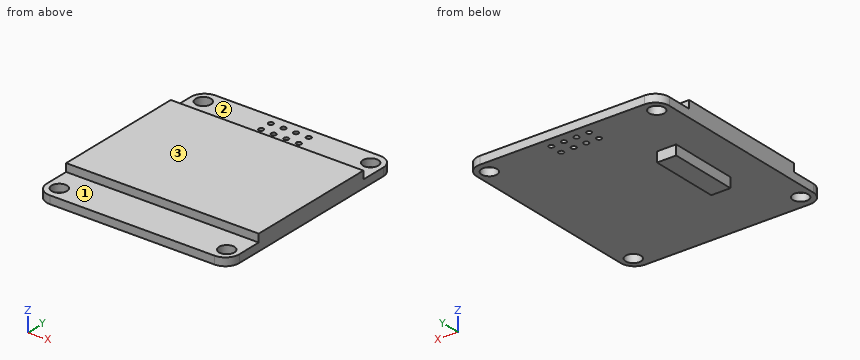
from build123d import *

# Parameters (mm, degrees)
SKIZZE1_R                       = 1.55
AUFSATZ_LINEAR_AUSTRAGEN1_DEPTH = 1.6
SKIZZE2_R                       = 0.5
SCHNITT_LINEAR_AUSTRAGEN1_DEPTH = 1.6
SKIZZE3_W                       = 38.8
SKIZZE3_H                       = 27.043851976
AUFSATZ_LINEAR_AUSTRAGEN2_DEPTH = 1.6
SKIZZE4_W                       = 3.86922581
SKIZZE4_H                       = 14.010670301
AUFSATZ_LINEAR_AUSTRAGEN3_DEPTH = 2


with BuildPart() as part:
    # Skizze1 → Aufsatz-Linear austragen1 (new body)
    with BuildSketch(Plane.XY):
        with BuildLine():
            Line((16.6, -21.4), (-16.6, -21.4))
            ThreePointArc((-16.6, -21.4), (-18.579898987, -20.579898987), (-19.4, -18.6))
            Line((-19.4, -18.6), (-19.4, 18.6))
            ThreePointArc((-19.4, 18.6), (-18.579898987, 20.579898987), (-16.6, 21.4))
            Line((-16.6, 21.4), (16.6, 21.4))
            ThreePointArc((16.6, 21.4), (18.579898987, 20.579898987), (19.4, 18.6))
            Line((19.4, 18.6), (19.4, -18.6))
            ThreePointArc((19.4, -18.6), (18.579898987, -20.579898987), (16.6, -21.4))
        make_face()
        with Locations((-16.861682243, 18.6)):
            Circle(SKIZZE1_R, mode=Mode.SUBTRACT)
        with Locations((-16.861682243, -18.6)):
            Circle(SKIZZE1_R, mode=Mode.SUBTRACT)
        with Locations((16.861682243, -18.6)):
            Circle(SKIZZE1_R, mode=Mode.SUBTRACT)
        with Locations((16.861682243, 18.6)):
            Circle(SKIZZE1_R, mode=Mode.SUBTRACT)
    extrude(amount=AUFSATZ_LINEAR_AUSTRAGEN1_DEPTH)

    # Skizze2 → Schnitt-Linear austragen1 (cut)
    with BuildSketch(Plane.XY.offset(1.6)):
        with Locations((-3.81, 16.782506105)):
            Circle(SKIZZE2_R)
        with Locations((-1.27, 16.782506105)):
            Circle(SKIZZE2_R)
        with Locations((1.27, 16.782506105)):
            Circle(SKIZZE2_R)
        with Locations((3.81, 16.782506105)):
            Circle(SKIZZE2_R)
        with Locations((-1.27, 19.322506105)):
            Circle(SKIZZE2_R)
        with Locations((1.27, 19.322506105)):
            Circle(SKIZZE2_R)
        with Locations((3.81, 19.322506105)):
            Circle(SKIZZE2_R)
        with Locations((-3.81, 19.322506105)):
            Circle(SKIZZE2_R)
    extrude(amount=-SCHNITT_LINEAR_AUSTRAGEN1_DEPTH, mode=Mode.SUBTRACT)

    # Skizze3 → Aufsatz-Linear austragen2 (add)
    with BuildSketch(Plane.XY.offset(1.6)):
        with Locations((0, -0.061093039)):
            Rectangle(SKIZZE3_W, SKIZZE3_H)
    extrude(amount=AUFSATZ_LINEAR_AUSTRAGEN2_DEPTH)

    # Skizze4 → Aufsatz-Linear austragen3 (add)
    with BuildSketch(Plane(origin=(0, 0, 0), x_dir=(-1, 0, 0), z_dir=(0, 0, -1))):
        with Locations((10.304359262, 0.631294738)):
            Rectangle(SKIZZE4_W, SKIZZE4_H)
    extrude(amount=AUFSATZ_LINEAR_AUSTRAGEN3_DEPTH)


solid = part.part
The model under review builds one solid part; all positions refer to its coordinate system, in mm. Face numbers are marked on the shaded views. A direction names the side the tool comes from. Round coordinates to 2 decimals unless told otherwise and drop trailing zeros. Order: outer loops, then holes, each group sorted by start corner. A loop starts at its lowest first (then second) coordinate and runs counter-clockwise, first axis right, second up. Notation, with made-up numbers: (84, -9) -> (131, -9) arc R20 cw to (131, 0) -> close; hole circle Ø9 at (73, -23). An arc over 180 degrees is marked (long way). Write item = value, one per line. Start each with the question number.
Item 1: For the marked faces 1, 2 and 3, list the 3-axis set-ups (+Z, -Z, +X, -X, +Y, -Y) from which the entire face can be reached by the end or side of a thin tool; tool diameter is ignored.
Item 2: Consider section D-D on x = 16. Write out the cut boundary in (y, z), plus the area to 3 significant figures.
Item 3: Clearance check with flat-ended pins moving along their axes: pin 1 Ø1.5 at (x, z) = (3, 2.5) entering from +Y; pin 2 Ø2 at (x, y) = (7, -15) entering from +Z; pin 3 Ø2 at (x, z) = (-10.5, -0.5) entering from +Y; pin 4 Ø19.5 at (x, y) = (5.5, -10.5) entering from -Z. State where each tip first meets the part, or that it passes through.
Item 4: Consider section C-C on x = -14. Write out the cut boundary in (y, z), plus the area to 3 significant figures.
Item 5: Consider section A-A on x = 1.27. Write out the cut boundary in (y, z), plus the area to 3 significant figures.
Item 6: Consider section B-B on z = 0.7. Count the separate pieces of the cut face and the enclosed holes in it, plus the area to 3 significant figures.
Item 7: For line 1 along Y through (x, z) = (3.81, 0.95); line 2 along Z through (x, y) = (12.5, 9); line 3 along Z through (x, y) = (-15.5, -20), list the stretches that pass through material, from the lowest coordinate up.
Conclusion:
q1.face_1 = +Z, +X, -X, -Y
q1.face_2 = +Z, +X, -X, +Y
q1.face_3 = +Z, +X, -X, +Y, -Y
q2.outline = (-21.4, 0) -> (-19.89, 0) -> (-19.89, 1.6) -> (-21.4, 1.6) -> close; (-17.31, 0) -> (17.31, 0) -> (17.31, 1.6) -> (13.46, 1.6) -> (13.46, 3.2) -> (-13.58, 3.2) -> (-13.58, 1.6) -> (-17.31, 1.6) -> close; (19.89, 0) -> (21.4, 0) -> (21.4, 1.6) -> (19.89, 1.6) -> close
q2.area = 104 mm2
q3.pin_1 = 13.46
q3.pin_2 = 1.6
q3.pin_3 = 21.4
q3.pin_4 = 0
q4.outline = (-21.4, 0) -> (21.4, 0) -> (21.4, 1.6) -> (13.46, 1.6) -> (13.46, 3.2) -> (-13.58, 3.2) -> (-13.58, 1.6) -> (-21.4, 1.6) -> close
q4.area = 112 mm2
q5.outline = (-21.4, 0) -> (16.28, 0) -> (16.28, 1.6) -> (13.46, 1.6) -> (13.46, 3.2) -> (-13.58, 3.2) -> (-13.58, 1.6) -> (-21.4, 1.6) -> close; (17.28, 0) -> (18.82, 0) -> (18.82, 1.6) -> (17.28, 1.6) -> close; (19.82, 0) -> (21.4, 0) -> (21.4, 1.6) -> (19.82, 1.6) -> close
q5.area = 109 mm2
q6.separate_pieces = 1
q6.enclosed_holes = 12
q6.area = 1,620 mm2
q7.line_1 = -21.4 to 16.28, 17.28 to 18.82, 19.82 to 21.4
q7.line_2 = 0 to 3.2
q7.line_3 = 0 to 1.6
